Geometry check sheet. Reference: the model listing, model coordinates, mm. Face numbers are marked on the shaded views. Give positions to 0.01 mm unless a question says otherwise; leave off trailing zeros. Loops run counter-clockwise (first coordinate to the right, second up) from the corner with the lowest first, then second, coordinate; pieces in that order, holes last.
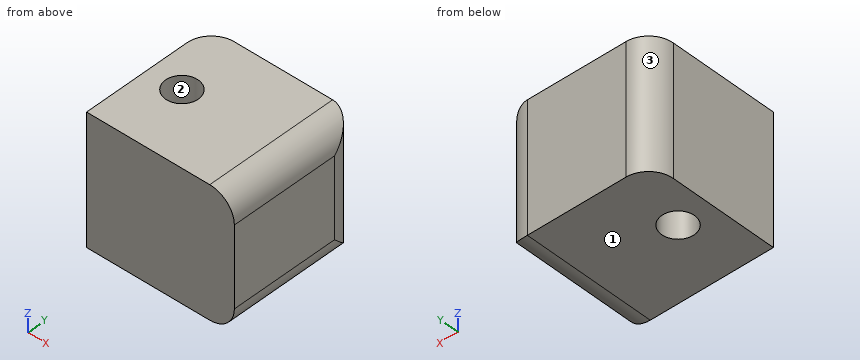
Autodesk Inventor part; units mm, degrees
ref_plane "YZ Plane" through (0, 0, 0) normal (1, 0, 0) x (0, 1, 0)
ref_plane "XZ Plane" through (0, 0, 0) normal (0, 1, 0) x (-1, 0, 0)
ref_plane "XY Plane" through (0, 0, 0) normal (0, 0, 1) x (1, 0, 0)
sketch "Эскиз2" plane through (0, 0, 0) normal (0, 1, 0) x (-1, 0, 0)
  line L0 (5.5, 5.25) -> (-5.5, 5.25)
  line L1 (-5.5, 5.25) -> (-5.5, -5.25)
  line L2 (-5.5, -5.25) -> (5.5, -5.25)
  line L3 (5.5, -5.25) -> (5.5, 5.25)
  line L4 (5.5, 0) -> (-5.5, 0) construction
  line L5 (0, 5.25) -> (0, -5.25) construction
  circle A0 centre (0, 0) radius 1.25
  line L6 (-5.5, -5.25) -> (-6.5, -5.25)
  line L7 (-6.5, -5.25) -> (-6.5, 5.25)
  line L8 (-6.5, 5.25) -> (-5.5, 5.25)
  line L9 (-5.5, 5.25) -> (-5.5, -5.25)
  dimension "d0" = 11
  dimension "d1" = 10.5
  dimension "d2" = 2.5
  dimension "d12" = 1
extrude "Выдавливание1" add sketch "Эскиз2" along normal blind 10.8 contours L3 L2 L1 L0 | L1 L6 L7 L8 | A0
sketch "Эскиз4" plane through (-5.5, 0, 5.25) normal (0, 0, 1) x (1, 0, 0)
  line L0 (5.5, 0) -> (2.75, 10.8) construction
  line L1 (5.5, 10.8) -> (0, 10.8) construction
  line L2 (0, 0) -> (0, 10.8) construction
  line L3 (0, 5.4) -> (5.5, 5.4) construction
  line L4 (5.5, 0) -> (5.5, 10.8) construction
  circle A0 centre (2.75, 5.4) radius 1.325
  dimension "d8" = 2.65
extrude "Выдавливание3" cut sketch "Эскиз4" against normal blind 10.5
fillet "Сопряжение2" radius 2 4 edges at (6.5, 5.4, 5.25) (6.5, 5.4, -5.25) (6.5, 10.8, 0) (-5.5, 10.8, 0)
properties part number "pusher"
1) Sectioned sample at A-A on y = 5.4. Enter the section's corners in (x, z) (3 decimals).
2) Scan lines: line 1 along Y through (x, z) = (-2.75, -2) (3 decimals); line 2 along X through (y, z) = (5.25, 0); line 3 along Z through (x, y) = (5.75, 10). Record each from-to range of solid material in increasing order.
3) Sectioned sample at C-C on z = 1.25. Enter the section's corners in (x, y) (3 decimals), plus the area to 3 significant figures.
4) Mould release check, pull along Y, two halves, no side actions. Record for the marked faces 1, 2 and 3: +Y half, -Y half, draft (parallel to the pull), parting line (faces both ways), or undercut.
5) Sectioned sample at B-B on x = -2.75. Enter the section's corners in (y, z) (3 decimals).
6) Depth check by flat-ended pin: P1, Ø2.5, axis at x = -2.75, y = 5.4, coming from the -Z side. Enter the tip coordinate at first touch or a pass-through.
7) Sectioned sample at D-D on z = 4. Enter the section's corners in (x, y) (3 decimals).
Determined:
1. outline: (-5.5, -5.25) - (-4.075, -5.25) - (-4.075, 5.25) - (-5.5, 5.25) - close; (-1.425, -5.25) - (4.5, -5.25) arc R2 ccw to (6.5, -3.25) - (6.5, 3.25) arc R2 ccw to (4.5, 5.25) - (-1.425, 5.25) - close
2. line 1: y = 0 to 4.075, 6.725 to 10.8
2. line 2: x = -5.5 to -4.07, -1.43 to 6.5
2. line 3: z = -4.81 to 4.81
3. outline: (-5.5, 0) - (6.5, 0) - (6.5, 8.8) arc R2 ccw to (4.5, 10.8) - (-3.5, 10.8) arc R2 ccw to (-5.5, 8.8) - close; hole circle Ø2.65 at (-2.75, 5.4)
3. area: 122 mm2
4. face 1: draft
4. face 2: undercut
4. face 3: +Y half
5. outline: (0, -5.25) - (4.075, -5.25) - (4.075, 5.25) - (0, 5.25) - close; (6.725, -5.25) - (10.8, -5.25) - (10.8, 5.25) - (6.725, 5.25) - close
6. P1: passes through
7. outline: (-5.5, 0) - (6.354, 0) - (6.354, 9.55) arc R2 ccw to (4.5, 10.8) - (-3.5, 10.8) arc R2 ccw to (-5.5, 8.8) - close; hole circle Ø2.65 at (-2.75, 5.4)
